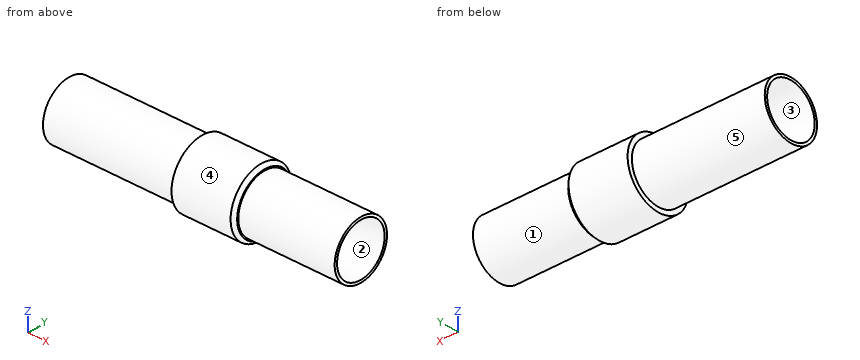
from build123d import *

# Parameters (mm, degrees)
SKETCH_2_R      = 32
SKETCH_2_R_2    = 27.5
EXTRUDE_1_DEPTH = 60
CHAMFER_1_SIZE  = 3.2875


with BuildPart() as part:
    # Эскиз1 → Повернуть1 (revolve)
    with BuildSketch(Plane.XY):
        Polygon((0, 27.5), (-280, 27.5), (-280, 25), (-145, 12.5), (-77.5, 12.5), (0, 25), align=None)
    revolve(axis=Axis((0, 0, 0), (-1, 0, 0)))

    # Эскиз2 → Бобышка-Вытянуть1 (add)
    with BuildSketch(Plane(origin=(-152.5, 0, 0), x_dir=(0, 0, -1), z_dir=(1, 0, 0))):
        Circle(SKETCH_2_R)
        Circle(SKETCH_2_R_2, mode=Mode.SUBTRACT)
    extrude(amount=EXTRUDE_1_DEPTH)

    # Фаска1
    chamfer_1_edges = [part.edges().sort_by_distance(p)[0] for p in [
        (-92.5, 0, 32),
    ]]
    chamfer(chamfer_1_edges, length=CHAMFER_1_SIZE)


solid = part.part
The listing builds one solid part. Answer for the finished solid, in the listing's coordinates (mm). Face numbers are marked on the shaded views. A direction names the side the tool comes from. Coordinates: 2 decimals unless noted, no trailing zeros. Order: outer loops, then holes, each group sorted by start corner. A loop starts at its lowest first (then second) coordinate and runs counter-clockwise, first axis right, second up.
Q1. Consider line 1 (Y direction, x = -97.5, z = 0); line 2 (Z direction, x = -253.5, y = 14); line 3 (Y direction, x = -116, z = -11). Determine where each line is inside the solid, lowest interval first.
Q2. A cutting plane is placed at D-D, the plane x = -85. Write down the section's boundary in (y, z).
Q3. Which of the six approach directions +Z, -Z, +X, -X, +Y, -Y give full straight-line access (tool end or side, diameter ignored) to the marked faces 4 and 5?
Q4. For a pull along Z with two mould halves and no side action, classify the marked faces 1, 2 and 3 as pulls with the +Z half, pulls with the -Z half, needs draft (parallel to the pull), parting line crosses it, or undercut.
Q5. A cutting plane is placed at A-A, the plane y = 0. Write down the section's boundary in (x, z), and give its area (3 significant figures).
Q6. A cutting plane is placed at C-C, the plane x = -164.5. Write down the section's boundary in (y, z).
Q7. Given P1, Ø2, axis at x = -97.5, y = 18, coming from the -Z side; P2, Ø4, axis at x = -197.5, z = 17.5, coming from the -Y side; P3, Ø6, axis at x = -118.5, y = -8.5, coming from the -Z side, each flat-ended and moving along its own axis, determine where each tip first touches the part or whether it passes through.
Answers follow:
1. line 1: y = -32 to -12.5, 12.5 to 32
1. line 2: z = -23.67 to -17.67, 17.67 to 23.67
1. line 3: y = -30.05 to -5.94, 5.94 to 30.05
2. outline: circle Ø55 at (0, 0); hole circle Ø25 at (0, 0)
3. face 4: +X, -X
3. face 5: -X
4. face 1: parting line crosses it
4. face 2: undercut
4. face 3: undercut
5. outline: (-280, -27.5) - (-152.5, -27.5) - (-152.5, -32) - (-95.79, -32) - (-92.5, -28.71) - (-92.5, -27.5) - (0, -27.5) - (0, -25) - (-77.5, -12.5) - (-145, -12.5) - (-280, -25) - close; (-280, 25) - (-145, 12.5) - (-77.5, 12.5) - (0, 25) - (0, 27.5) - (-92.5, 27.5) - (-92.5, 28.71) - (-95.79, 32) - (-152.5, 32) - (-152.5, 27.5) - (-280, 27.5) - close
5. area: 6,270 mm2
6. outline: circle Ø55 at (0, 0); hole circle Ø28.61 at (0, 0)
7. P1: stops at z = -27.11
7. P2: stops at y = -22.72
7. P3: stops at z = -31.52
